```python
from build123d import *
from OCP.BRepFilletAPI import BRepFilletAPI_MakeChamfer

# Parameters (mm, degrees)
SKETCH2_W           = 100
SKETCH2_H           = 50
SKETCH2_W_2         = 91
SKETCH2_H_2         = 40
BOSS_EXTRUDE1_DEPTH = 10
SKETCH3_W           = 100
SKETCH3_H           = 50
BOSS_EXTRUDE2_DEPTH = 5
CHAMFER1_SIZE       = 17
CHAMFER1_SIZE_2     = 2.997558672
CHAMFER2_SIZE       = 1
CHAMFER2_SIZE2      = 1.031574872


with BuildPart() as part:
    # Sketch2 → Boss-Extrude1 (new body)
    with BuildSketch(Plane(origin=(0, 0, 0), x_dir=(1, 0, 0), z_dir=(0, 1, 0))):
        Rectangle(SKETCH2_W, SKETCH2_H)
        Rectangle(SKETCH2_W_2, SKETCH2_H_2, mode=Mode.SUBTRACT)
    extrude(amount=BOSS_EXTRUDE1_DEPTH)

    # Sketch3 → Boss-Extrude2 (add)
    with BuildSketch(Plane.XZ):
        Rectangle(SKETCH3_W, SKETCH3_H)
    extrude(amount=BOSS_EXTRUDE2_DEPTH)

    # Chamfer1
    # the kernel refuses this chamfer: 17, 2.997558672 mm, written as the material it takes off along each edge
    with BuildSketch(Plane(origin=(-50, 10, 69.175159539), x_dir=(-0.0066825316561016975, -0.9999776716360548, 0), z_dir=(0, 0, -1)), Plane(origin=(50, 10, -69.175159539), x_dir=(0.0066825316561016975, -0.9999776716360548, 0), z_dir=(0, 0, 1))) as chamfer1_piece_1:
        Polygon((CHAMFER1_SIZE * 0.999977671636, -CHAMFER1_SIZE * 0.0066825316561), (-CHAMFER1_SIZE_2 * 0.0066825316562, -CHAMFER1_SIZE_2 * 0.999977671651), (0, 0), align=None)
    extrude(amount=138.350319078, mode=Mode.SUBTRACT)
    with BuildSketch(Plane(origin=(-94.175159539, 10, -25), x_dir=(0, -0.9999776716360548, -0.0066825316561016975), z_dir=(1, 0, 0)), Plane(origin=(94.175159539, 10, 25), x_dir=(0, -0.9999776716360548, 0.0066825316561016975), z_dir=(-1, 0, 0))) as chamfer1_piece_2:
        Polygon((CHAMFER1_SIZE * 0.999977671636, -CHAMFER1_SIZE * 0.0066825316561), (-CHAMFER1_SIZE_2 * 0.0066825316562, -CHAMFER1_SIZE_2 * 0.999977671651), (0, 0), align=None)
    extrude(amount=188.350319078, mode=Mode.SUBTRACT)

    # Chamfer2: one chamfer whose edges measure the first distance from different faces: ONE call of the kernel's chamfer builder (chamfer() names one face for all edges)
    chamfer2_edges_1 = [part.edges().sort_by_distance(p)[0] for p in [
        (48.324893683, 2.5, -23.324893683),
        (48.324893683, 2.5, 23.324893683),
    ]]
    chamfer2_side_1 = [part.faces().sort_by_distance(p)[0] for p in [
        (48.349886727, 2.358257408, 0),
    ]]
    chamfer2_edges_2 = [part.edges().sort_by_distance(p)[0] for p in [
        (-48.324893683, 2.5, -23.324893683),
    ]]
    chamfer2_side_2 = [part.faces().sort_by_distance(p)[0] for p in [
        (0, 2.431585346, -23.336957033),
    ]]
    chamfer2_edges_3 = [part.edges().sort_by_distance(p)[0] for p in [
        (-48.324893683, 2.5, 23.324893683),
    ]]
    chamfer2_side_3 = [part.faces().sort_by_distance(p)[0] for p in [
        (0, 2.431585346, 23.336957033),
    ]]
    chamfer2 = BRepFilletAPI_MakeChamfer(part.part.solid().wrapped)
    for e in chamfer2_edges_1:
        chamfer2.Add(CHAMFER2_SIZE, CHAMFER2_SIZE2, e.wrapped, chamfer2_side_1[0].wrapped)  # the first distance lies on this face
    for e in chamfer2_edges_2:
        chamfer2.Add(CHAMFER2_SIZE, CHAMFER2_SIZE2, e.wrapped, chamfer2_side_2[0].wrapped)  # the first distance lies on this face
    for e in chamfer2_edges_3:
        chamfer2.Add(CHAMFER2_SIZE, CHAMFER2_SIZE2, e.wrapped, chamfer2_side_3[0].wrapped)  # the first distance lies on this face
    add(Compound.cast(chamfer2.Shape()), mode=Mode.REPLACE)


solid = part.part
```
Build history of the part. All positions in model axes, mm. A direction names the side the tool comes from. Round coordinates to 2 decimals unless told otherwise and drop trailing zeros. Write each loop counter-clockwise with the first axis right and the second up, starting at its lowest first coordinate (ties: lowest second). Pieces come first, ordered by that corner, then holes. Notation, with made-up numbers: (-6.75, 44.5) - (5.25, 44.5) arc R17 cw to (5.25, 59.5) - close; hole circle Ø6 at (89.5, 52). An arc over 180 degrees is marked (long way). Answer as CSV lines item,"result".
Q1. Tool access for faces 4 (the flat face through (0, 10, -21)), 5 (the flat face through (-1, 0, 0)): list every direction of +Z, -Z, +X, -X, +Y, -Y with a clear straight run to the whole face (end or side of a thin tool).
Report:
face 4,"+Z, -Z, +X, -X, +Y"
face 5,"+Y"
Q2. Drill centre lines: probe 1 along Y at (x, z) = (-3.5, 8); probe 2 along X at (y, z) = (8.25, -10); probe 3 along Z at (x, y) = (30, 4). Where is each one in solid material? Low to high. Write a range as [from, to].
Report:
probe 1,"y = [-5, 0]"
probe 2,"x = [-47.31, -45.5], [45.5, 47.31]"
probe 3,"z = [-23.06, -20], [20, 23.06]"
Q3. Cut at C-C (x = 41). Write the cut outline in (y, z), and give its area (3 significant figures).
Report:
outline,"(-5, -24.65) - (10, -22) - (10, -20) - (0, -20) - (0, 20) - (10, 20) - (10, 22) - (-5, 24.65) - close"
area,"300 mm^2"
Q4. Cut at A-A (z = 4). Write the cut outline in (x, y), and give its area (3 significant figures).
Report:
outline,"(-49.65, -5) - (49.65, -5) - (47, 10) - (45.5, 10) - (45.5, 0) - (-45.5, 0) - (-45.5, 10) - (-47, 10) - close"
area,"540 mm^2"
Q5. Pull direction Z, two halves, no side cores. Call faces 1 (the flat face through (-1, 5, -20)), 2 (the flat face through (-48.343, 2.395, 0.33)), 3 (the flat face through (-0.697, 2.395, -23.343)): +Z half, -Z half, draft (parallel to the pull), parting line (faces both ways), or undercut.
Report:
face 1,"undercut"
face 2,"draft"
face 3,"-Z half"
Q6. Cut at B-B (y = 1.25). Write the cut outline in (x, z).
Report:
outline,"(-48.55, -22.5) - (-47.53, -23.55) - (47.5, -23.55) - (48.55, -22.53) - (48.55, 22.53) - (47.5, 23.55) - (-47.53, 23.55) - (-48.55, 22.5) - close; hole (-45.5, -20) - (45.5, -20) - (45.5, 20) - (-45.5, 20) - close"
Q7. Cut at D-D (y = 7). Write the cut outline in (x, z).
Report:
outline,"(-47.53, -21.48) - (-46.52, -22.53) - (46.48, -22.53) - (47.53, -21.52) - (47.53, 21.52) - (46.48, 22.53) - (-46.52, 22.53) - (-47.53, 21.48) - close; hole (-45.5, -20) - (45.5, -20) - (45.5, 20) - (-45.5, 20) - close"
Q8. Drop flat-ended pins along their axis: pin 1 (5 mm diameter, centred on x = -36, z = 7, fed in from +Y); pin 2 (5 mm diameter, centred on x = 1, y = 3, fed in from +Z); pin 3 (3 mm diameter, centred on x = -32, y = -1.5, fed in from -Z). Give the stop position or say it passes through.
Report:
pin 1,"stops at y = 0"
pin 2,"stops at z = 23.68"
pin 3,"stops at z = -24.29"
